Verification items for the finished model (mm, model axes). A direction names the side the tool comes from. Give positions to 0.01 mm unless a question says otherwise; leave off trailing zeros. Write each loop counter-clockwise with the first axis right and the second up, starting at its lowest first coordinate (ties: lowest second). Pieces come first, ordered by that corner, then holes. Notation, with made-up numbers: (54, -23) - (97, -23) arc R19 ccw to (97, -15) - close; hole circle Ø3 at (-12.5, 32.25). An arc over 180 degrees is marked (long way). Answer as a JSON object with one key per item and string values. Group by question number.
Item 1: Scan lines: line 1 along Y through (x, z) = (3, 0.3); line 2 along X through (y, z) = (-2, 1.2); line 3 along X through (y, z) = (3.5, 0.4). Record each from-to range of solid material in increasing order. Write a range as [from, to].
Item 2: Sectioned sample at A-A, the plane y = 0. Record the boundary of the cut face in (x, z).
Item 3: Sectioned sample at B-B, the plane x = 0. Record the boundary of the cut face in (y, z).
Item 4: Sectioned sample at D-D, the plane x = 15.5. Record the boundary of the cut face in (y, z).
Item 5: Tool access check on faces 1 (the face through (0.01, 3.35, 0.76)), 2 (the face through (-13, 3, 0.5)), 3 (the face through (0, -5, 1.5)). Record the directions out of +Z, -Z, +X, -X, +Y, -Y that give a thin tool (end or side, any length) a straight path to the whole face; none if there is none.
Item 6: Go/stop test with flat-tipped pins: pin 1 (1.2 mm diameter, centred on x = 3, y = -11.5, fed in from -Z); pin 2 (1.2 mm diameter, centred on x = 8.5, y = 9, fed in from -Z). Record where each tip stops, or that it passes through.
Item 7: Sectioned sample at C-C, the plane z = 1.25. Record the boundary of the cut face in (x, y), and give its area (3 significant figures).
Item 8: Draft check along X on faces 4 (the face through (2.67, -9.64, 0.25)), 5 (the face through (23.846, 7.509, 0.74)), 6 (the face through (0, -5, 0)). Enter one of: +X half, -X half, draft (parallel to the pull), parting line (faces both ways), or undercut.
```python
from build123d import *

# Parameters (mm, degrees)
SKETCH_R              = 25
PAD_DEPTH             = 1.5
POCKET_DEPTH          = 1.5
POLARPATTERN_COUNT    = 3
SKETCH002_R           = 1
POCKET001_DEPTH       = 5
POLARPATTERN001_COUNT = 3
SKETCH003_R           = 2
POCKET002_DEPTH       = 0.5
POLARPATTERN002_COUNT = 3


with BuildPart() as part:
    # Sketch → Pad (new body)
    with BuildSketch(Plane.XY):
        Circle(SKETCH_R)
    extrude(amount=PAD_DEPTH)

    # Sketch001 (on Face3 of Pad) → Pocket (cut)
    with BuildSketch(Plane.XY.offset(1.5)):
        with BuildLine():
            ThreePointArc((-0.62801, 2.264532), (0, -2.35), (0.62801, 2.264532))
            Line((0.895249, 3.228162), (0.62801, 2.264532))
            ThreePointArc((0.895249, 3.228162), (0, 3.35), (-0.895249, 3.228162))
            Line((-0.895249, 3.228162), (-0.62801, 2.264532))
        make_face()
    pocket = extrude(amount=-POCKET_DEPTH, mode=Mode.SUBTRACT)

    # PolarPattern: Pocket ×3 about axis
    polarpattern_axis = Axis((0, 0, 1.5), (0, 0, 1))
    for i in range(1, POLARPATTERN_COUNT):
        add(pocket.rotate(polarpattern_axis, i * 360 / POLARPATTERN_COUNT), mode=Mode.SUBTRACT)

    # Sketch002 (on Face3 of PolarPattern) → Pocket001 (cut)
    with BuildSketch(Plane.XY.offset(1.5)):
        with Locations((8.485281, 8.485281)):
            Circle(SKETCH002_R)
    pocket001 = extrude(amount=-POCKET001_DEPTH, mode=Mode.SUBTRACT)

    # PolarPattern001: Pocket001 ×3 about axis
    polarpattern001_axis = Axis((0, 0, 1.5), (0, 0, 1))
    for i in range(1, POLARPATTERN001_COUNT):
        add(pocket001.rotate(polarpattern001_axis, i * 360 / POLARPATTERN001_COUNT), mode=Mode.SUBTRACT)

    # Sketch003 (on Face2 of PolarPattern001) → Pocket002 (cut)
    with BuildSketch(Plane(origin=(0, 0, 0), x_dir=(1, 0, 0), z_dir=(0, 0, -1))):
        with Locations((3.105829, 11.59111)):
            Circle(SKETCH003_R)
    pocket002 = extrude(amount=-POCKET002_DEPTH, mode=Mode.SUBTRACT)

    # PolarPattern002: Pocket002 ×3 about axis
    polarpattern002_axis = Axis((0, 0, 0), (0, 0, -1))
    for i in range(1, POLARPATTERN002_COUNT):
        add(pocket002.rotate(polarpattern002_axis, i * 360 / POLARPATTERN002_COUNT), mode=Mode.SUBTRACT)


solid = part.part
```
Geometry check:
{
 "1": {"line 1": "[-24.82, -13.59], [-9.59, -1.49], [-0.78, 24.82]", "line 2": "[-24.92, -2.69], [-1.97, -1.23], [1.23, 1.97], [2.69, 24.92]", "line 3": "[-24.75, -13.55], [-9.63, 24.75]"},
 "2": {"outline": "(-25, 0) - (-2.35, 0) - (-2.35, 1.5) - (-25, 1.5) - close; (2.35, 0) - (25, 0) - (25, 1.5) - (2.35, 1.5) - close"},
 "3": {"outline": "(-25, 0) - (-2.35, 0) - (-2.35, 1.5) - (-25, 1.5) - close; (3.35, 0) - (25, 0) - (25, 1.5) - (3.35, 1.5) - close"},
 "4": {"outline": "(-19.62, 0) - (19.62, 0) - (19.62, 1.5) - (-19.62, 1.5) - close"},
 "5": {"face 1": "+Z, -Z", "face 2": "-Z", "face 3": "+Z, +X, -X, +Y, -Y"},
 "6": {"pin 1": "through", "pin 2": "z = 0.5"},
 "7": {"outline": "circle Ø50 at (0, 0); hole circle Ø2 at (-11.59, 3.11); hole (-3.24, -0.84) arc R3.35 ccw to (-2.35, -2.39) - (-1.65, -1.68) arc R2.35 ccw to (1.65, -1.68) - (2.35, -2.39) arc R3.35 ccw to (3.24, -0.84) - (2.28, -0.59) arc R2.35 ccw to (0.63, 2.26) - (0.9, 3.23) arc R3.35 ccw to (-0.9, 3.23) - (-0.63, 2.26) arc R2.35 ccw to (-2.28, -0.59) - close; hole circle Ø2 at (3.11, -11.59); hole circle Ø2 at (8.49, 8.49)", "area": "1,930 mm^2"},
 "8": {"face 4": "undercut", "face 5": "parting line", "face 6": "draft"}
}
